Work out the finished part from the listing and answer in its coordinate system (mm). A direction names the side the tool comes from. Coordinates: 2 decimals unless noted, no trailing zeros. Write each loop counter-clockwise with the first axis right and the second up, starting at its lowest first coordinate (ties: lowest second). Pieces come first, ordered by that corner, then holes. Notation, with made-up numbers: (-30, 61) - (-1, 61) arc R25 cw to (-1, 85) - close; hole circle Ø8 at (55.25, 31). An arc over 180 degrees is marked (long way). Use a Markdown table: item, result. Add a question column.
(1) The part is cut by section D-D, the plane x = 7.5. Give the vertices of the cut face in (y, z).
(2) The part is cut by section C-C, the plane z = -7.5. Give the vertices of the cut face in (x, y).
(3) Find the intervals of material crossed by line 1 (Z direction, x = 26.5, y = 7); line 2 (X direction, y = 3, z = 30); line 3 (Z direction, x = -21.5, y = 5), in increasing order. Write a range as from..to.
(4) A tool of negligible diameter and unlimited length cuts with its end or side. For faces 3 (the face through (10, 2.4, -22)), 4 (the face through (0, 7, 56.5)), 5 (the face through (0, 10, -21)), 6 (the face through (0, 5, -22.5)), 7 (the face through (31, 6, 15.5)), from which of +Z, -Z, +X, -X, +Y, -Y can it reach the whole face along a straight path? Write none if from no direction.
(5) The part is cut by section B-B, the plane x = -13.5. Give the vertices of the cut face in (y, z).
(6) The part is cut by section A-A, the plane y = 7.75. Give the vertices of the cut face in (x, z).
(7) For a pull along X with two mould halves and no side action, classify faces 1 (the face through (0, 0, 17)), 2 (the face through (-9, 2.4, -22)) as released by +X, released by -X, zero draft, split by the parting line, or undercut.
(8) Given pin 1 Ø0.9 at (x, y) = (21.5, 11) entering from -Z; pin 2 Ø10 at (x, z) = (-2.5, 10) entering from +Y; pin 3 Ø18.5 at (x, z) = (26.5, -13) entering from +Y, each flat-ended and moving along its own axis, determine where each tip first touches the part or whether it passes through.
from build123d import *

# Parameters (mm, degrees)
SKETCH1_W           = 61
SKETCH1_H           = 41
BOSS_EXTRUDE1_DEPTH = 1
SKETCH2_W           = 65
SKETCH2_H           = 45
SKETCH2_W_2         = 61
SKETCH2_H_2         = 41
BOSS_EXTRUDE2_DEPTH = 10
SKETCH3_W           = 8
SKETCH3_H           = 2
SKETCH3_W_2         = 10
SKETCH3_W_3         = 2
SKETCH3_H_2         = 16
CUT_EXTRUDE1_DEPTH  = 7.6
SKETCH4_W           = 65
SKETCH4_H           = 1
BOSS_EXTRUDE3_DEPTH = 35
SKETCH5_W           = 65
SKETCH5_H           = 35
SKETCH5_W_2         = 63
SKETCH5_H_2         = 33
BOSS_EXTRUDE4_DEPTH = 12
CUT_EXTRUDE2_REACH  = 69.316
SKETCH6_W           = 18.450763423
SKETCH6_H           = 7.617543819


with BuildPart() as part:
    # Sketch1 → Boss-Extrude1 (new body)
    with BuildSketch(Plane(origin=(0, 0, 0), x_dir=(1, 0, 0), z_dir=(0, 1, 0))):
        Rectangle(SKETCH1_W, SKETCH1_H)
    extrude(amount=BOSS_EXTRUDE1_DEPTH)

    # Sketch2 → Boss-Extrude2 (add)
    with BuildSketch(Plane.XZ):
        Rectangle(SKETCH2_W, SKETCH2_H)
        Rectangle(SKETCH2_W_2, SKETCH2_H_2, mode=Mode.SUBTRACT)
    extrude(amount=-BOSS_EXTRUDE2_DEPTH)

    # Sketch3 → Cut-Extrude1 (cut)
    with BuildSketch(Plane(origin=(0, 10, 0), x_dir=(1, 0, 0), z_dir=(0, 1, 0))):
        with Locations((-8.5, 21.5)):
            Rectangle(SKETCH3_W, SKETCH3_H)
        with Locations((10.5, 21.5)):
            Rectangle(SKETCH3_W_2, SKETCH3_H)
        with Locations((31.5, -7.5)):
            Rectangle(SKETCH3_W_3, SKETCH3_H_2)
    extrude(amount=-CUT_EXTRUDE1_DEPTH, mode=Mode.SUBTRACT)

    # Sketch4 → Boss-Extrude3 (add)
    with BuildSketch(Plane.XY.offset(22.5)):
        with Locations((0, 0.5)):
            Rectangle(SKETCH4_W, SKETCH4_H)
    extrude(amount=BOSS_EXTRUDE3_DEPTH)

    # Sketch5 → Boss-Extrude4 (add)
    with BuildSketch(Plane(origin=(0, 1, 0), x_dir=(1, 0, 0), z_dir=(0, 1, 0))):
        with Locations((0, -40)):
            Rectangle(SKETCH5_W, SKETCH5_H)
        with Locations((0, -40)):
            Rectangle(SKETCH5_W_2, SKETCH5_H_2, mode=Mode.SUBTRACT)
    extrude(amount=BOSS_EXTRUDE4_DEPTH)

    # Cut-Extrude2: up to this face of the body (flat: up to its plane)
    cut_extrude2_end = Plane(part.part.faces().sort_by_distance((0, 1, 40))[0])
    # Sketch6 → Cut-Extrude2 (cut, up to the picked face)
    with BuildSketch(Plane(origin=(0, 13, 0), x_dir=(1, 0, 0), z_dir=(0, 1, 0)), mode=Mode.PRIVATE) as cut_extrude2_sk1:
        with Locations((-16.202920441, -19.691228091)):
            Rectangle(SKETCH6_W, SKETCH6_H)
    cut_extrude2_tool1 = split(extrude(cut_extrude2_sk1.sketch, amount=-CUT_EXTRUDE2_REACH, mode=Mode.PRIVATE), bisect_by=cut_extrude2_end, keep=Keep.BOTH, mode=Mode.PRIVATE)
    add(cut_extrude2_tool1.solids().sort_by(Axis((-16.20292, 13, 19.691228), (0, -1, 0)))[0], mode=Mode.SUBTRACT)


solid = part.part
Model answer:
| question | item | result |
|---|---|---|
| 1 | outline | (0, -22.5) - (2.4, -22.5) - (2.4, -20.5) - (1, -20.5) - (1, 20.5) - (10, 20.5) - (10, 22.5) - (13, 22.5) - (13, 23.5) - (1, 23.5) - (1, 56.5) - (13, 56.5) - (13, 57.5) - (0, 57.5) - close |
| 2 | outline | (-32.5, 0) - (32.5, 0) - (32.5, 10) - (30.5, 10) - (30.5, 1) - (-30.5, 1) - (-30.5, 10) - (-32.5, 10) - close |
| 3 | line 1 | -22.5..-20.5, 20.5..23.5, 56.5..57.5 |
| 3 | line 2 | -32.5..-31.5, 31.5..32.5 |
| 3 | line 3 | -22.5..-20.5, 56.5..57.5 |
| 4 | face 3 | -Z, +Y |
| 4 | face 4 | +Y |
| 4 | face 5 | -Z, +X, -X, +Y |
| 4 | face 6 | -Z, +X, -X, +Y, -Y |
| 4 | face 7 | +X, +Y |
| 5 | outline | (0, -22.5) - (10, -22.5) - (10, -20.5) - (1, -20.5) - (1, 56.5) - (13, 56.5) - (13, 57.5) - (0, 57.5) - close |
| 6 | outline | (-32.5, -22.5) - (-12.5, -22.5) - (-12.5, -20.5) - (-30.5, -20.5) - (-30.5, 20.5) - (-25.43, 20.5) - (-25.43, 23.5) - (-31.5, 23.5) - (-31.5, 56.5) - (31.5, 56.5) - (31.5, 23.5) - (-6.98, 23.5) - (-6.98, 20.5) - (30.5, 20.5) - (30.5, 15.5) - (32.5, 15.5) - (32.5, 57.5) - (-32.5, 57.5) - close; (-4.5, -22.5) - (5.5, -22.5) - (5.5, -20.5) - (-4.5, -20.5) - close; (15.5, -22.5) - (32.5, -22.5) - (32.5, -0.5) - (30.5, -0.5) - (30.5, -20.5) - (15.5, -20.5) - close |
| 7 | face 1 | zero draft |
| 7 | face 2 | undercut |
| 8 | pin 1 | z = 22.5 |
| 8 | pin 2 | y = 1 |
| 8 | pin 3 | y = 10 |
